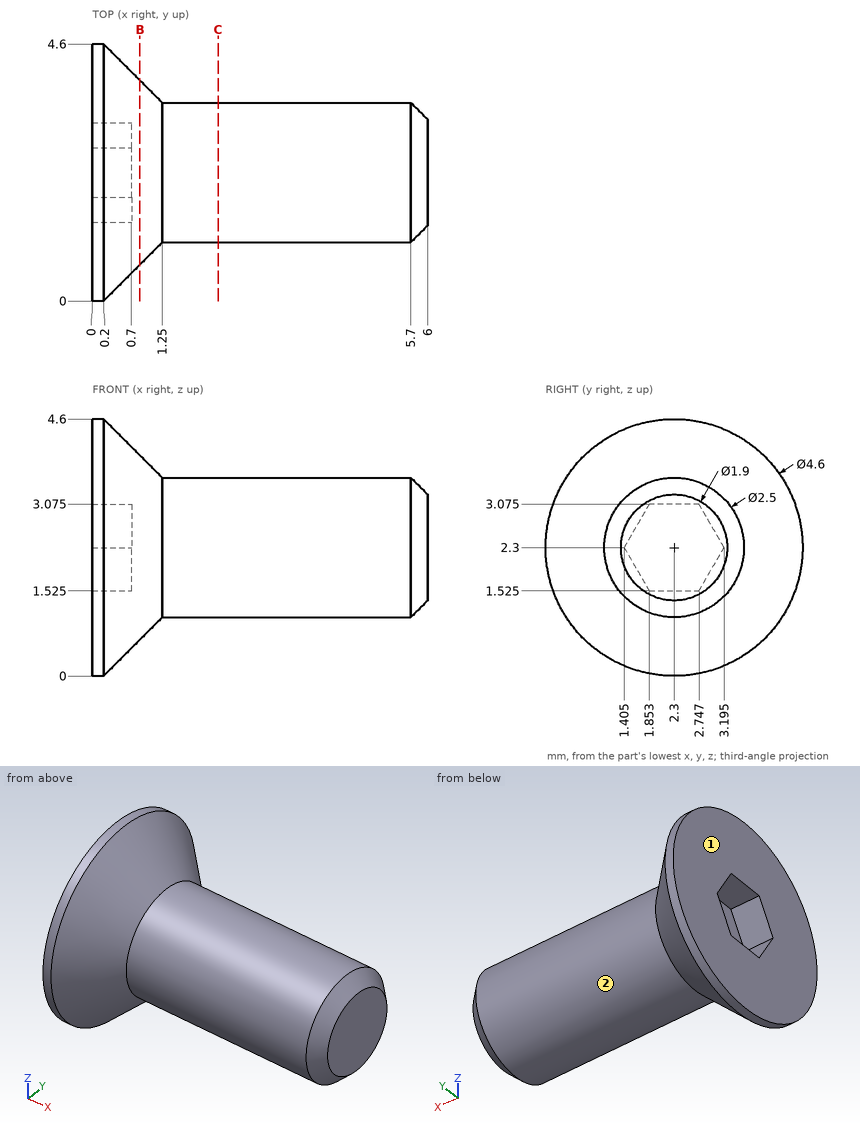
Check sheet for the drawn part. Datum: minimum x, y, z corner. Units: mm. A direction names the side the tool comes from. Round coordinates to 2 decimals unless told otherwise and drop trailing zeros. Order: outer loops, then holes, each group sorted by start corner. A loop starts at its lowest first (then second) coordinate and runs counter-clockwise, first axis right, second up. Notation, with made-up numbers: (67, 4) -> (91, 4) arc R22 cw to (91, 34) -> close; hole circle Ø11 at (9.25, -16.5). An arc over 180 degrees is marked (long way). Return JSON: item names as keys, results as strings. Group by question number.
Q1. Tool access check on the marked faces 1 and 2. Record the directions out of +Z, -Z, +X, -X, +Y, -Y that give a thin tool (end or side, any length) a straight path to the whole face; none if there is none.
Q2. Section check B-B, the plane x = 0.85. Record the boundary of the cut face in (y, z).
Q3. Material ranges on probe 1 along Y at (x, z) = (0.45, 2.7) (1 decimal); probe 2 along Y at (x, z) = (5.3, 1.95); probe 3 along Y at (x, z) = (0.55, 0.7) (1 decimal), recorded low to high. Write a range as from..to.
Q4. Section check C-C, the plane x = 2.25. Record the boundary of the cut face in (y, z).
Q5. Gauge pin test, flat ends, axial feed: pin 1 (1.5 mm diameter, centred on x = 5, z = 2.5, fed in from +Y); pin 2 (0.5 mm diameter, centred on y = 2.5, z = 2.5, fed in from -X); pin 3 (1 mm diameter, centred on x = 5, z = 1, fed in from -Y). Record the tip position at first contact, or that the pin passes through.
Numbers:
{
 "1": {"face 1": "+Z, -Z, -X, +Y, -Y", "face 2": "+X"},
 "2": {"outline": "circle Ø3.3 at (2.3, 2.3)"},
 "3": {"probe 1": "0.3..1.6, 3..4.3", "probe 2": "1.1..3.5", "probe 3": "1.2..3.4"},
 "4": {"outline": "circle Ø2.5 at (2.3, 2.3)"},
 "5": {"pin 1": "y = 3.55", "pin 2": "x = 0.7", "pin 3": "y = 1.34"}
}
